from build123d import *

# Parameters (mm, degrees)
BOSS_EXTRUDE1_DEPTH = 4
SKETCH2_R           = 2
SKETCH2_R_2         = 1.5
CUT_EXTRUDE1_DEPTH  = 95.026591983
SKETCH4_W           = 20
SKETCH4_H           = 100
BOSS_EXTRUDE2_DEPTH = 4
FILLET3_R           = 42
FILLET4_R           = 12
SKETCH7_R           = 2
CUT_EXTRUDE3_DEPTH  = 105.120122935
CHAMFER1_SIZE       = 10
FILLET8_R           = 2
CUT_EXTRUDE4_DEPTH  = 105.120122935
CUT_EXTRUDE5_DEPTH  = 105.120122935
SKETCH10_W          = 4
SKETCH10_H          = 14.148423286
CUT_EXTRUDE6_DEPTH  = 105.120122935
FILLET11_R          = 3
FILLET12_R          = 3


with BuildPart() as part:
    # Sketch1 → Boss-Extrude1 (new body)
    with BuildSketch(Plane.XY):
        Polygon((-40, 60), (-25, 60), (-25, 52), (-15, 52), (-15, 0), (-21, 0), (-21, -50), (21, -50), (21, 0), (15, 0), (15, 52), (25, 52), (25, 60), (40, 60), (40, -60), (22, -60), (22, -85), (12, -85), (12, -60), (-12, -60), (-12, -85), (-22, -85), (-22, -60), (-40, -60), align=None)
    extrude(amount=BOSS_EXTRUDE1_DEPTH)

    # Sketch2 → Cut-Extrude1 (cut, through all)
    with BuildSketch(Plane(origin=(0, 0, 0), x_dir=(-1, 0, 0), z_dir=(0, 0, -1))):
        with Locations((-28.5, -32)):
            Circle(SKETCH2_R)
        with Locations((17, -56.5)):
            Circle(SKETCH2_R_2)
        with Locations((28.8, -32)):
            Circle(SKETCH2_R)
        with Locations((-17, -56.5)):
            Circle(SKETCH2_R_2)
    extrude(amount=-CUT_EXTRUDE1_DEPTH, mode=Mode.SUBTRACT)

    # Sketch4 → Boss-Extrude2 (add)
    with BuildSketch(Plane.XY.offset(4)):
        with Locations((-50, 10)):
            Rectangle(SKETCH4_W, SKETCH4_H)
        with Locations((50, 10)):
            Rectangle(SKETCH4_W, SKETCH4_H)
    extrude(amount=-BOSS_EXTRUDE2_DEPTH)

    # Fillet3
    # the kernel refuses this fillet: 42 mm, written as the material it takes off along each edge
    with BuildSketch(Plane(origin=(60, 60, 107.531396204), x_dir=(0, -1, 0), z_dir=(0, 0, -1))) as fillet3_piece_1:
        with BuildLine():
            CenterArc((41.412558482, 42), FILLET3_R, 189.594068227, 80.405931773)
            Line((0, 35), (-0.82825117, 34.86))
            ThreePointArc((-0.82825117, 34.86), (-0.84, 17.5), (-0.84, 0))
            Line((-0.84, 0), (0, -0.84))
            Line((0, -0.84), (41.412558482, -0.84))
            Line((41.412558482, -0.84), (41.412558482, 0))
        make_face()
    extrude(amount=211.062792409, mode=Mode.SUBTRACT)
    with BuildSketch(Plane(origin=(-60, 60, 107.531396204), x_dir=(1, 0, 0), z_dir=(0, 0, -1))) as fillet3_piece_2:
        with BuildLine():
            CenterArc((42, 41.412558482), FILLET3_R, 180, 80.405931773)
            Line((0, 41.412558482), (-0.84, 41.412558482))
            Line((-0.84, 41.412558482), (-0.84, 0))
            Line((-0.84, 0), (0, -0.84))
            ThreePointArc((0, -0.84), (17.5, -0.84), (34.86, -0.82825117))
            Line((34.86, -0.82825117), (35, 0))
        make_face()
    extrude(amount=211.062792409, mode=Mode.SUBTRACT)

    # Fillet4
    fillet4_edges = [part.edges().sort_by_distance(p)[0] for p in [
        (60, -40, 2),
        (-60, -40, 2),
    ]]
    fillet(fillet4_edges, radius=FILLET4_R)

    # Sketch7 → Cut-Extrude3 (cut, through all)
    with BuildSketch(Plane.XY):
        with Locations(Location((-55, -20, 0), (0, 0, 180))):
            Circle(SKETCH7_R)
        with Locations(Location((55, -20, 0), (0, 0, 180))):
            Circle(SKETCH7_R)
        with Locations(Location((-37, -20, 0), (0, 0, 180))):
            Circle(SKETCH7_R)
        with Locations(Location((37, -20, 0), (0, 0, 180))):
            Circle(SKETCH7_R)
    extrude(amount=CUT_EXTRUDE3_DEPTH, mode=Mode.SUBTRACT)

    # Chamfer1
    chamfer1_edges = [part.edges().sort_by_distance(p)[0] for p in [
        (-40, -60, 2),
        (40, -60, 2),
    ]]
    chamfer(chamfer1_edges, length=CHAMFER1_SIZE)

    # Fillet8
    fillet8_edges = [part.edges().sort_by_distance(p)[0] for p in [
        (-30, -60, 2),
        (-40, -50, 2),
        (30, -60, 2),
        (40, -50, 2),
        (40, -40, 2),
        (-40, -40, 2),
    ]]
    fillet(fillet8_edges, radius=FILLET8_R)

    # Sketch8 → Cut-Extrude4 (cut, through all)
    with BuildSketch(Plane(origin=(0, 0, 0), x_dir=(-1, 0, 0), z_dir=(0, 0, -1))):
        with BuildLine():
            ThreePointArc((-17.964817996, 17.438774634), (-30.770630407, 21.535466224), (-44.214817996, 21.375674028))
            ThreePointArc((-44.214817996, 21.375674028), (-45.841525426, 19.061841075), (-43.527692473, 17.435133644))
            ThreePointArc((-43.527692473, 17.435133644), (-31.363903701, 17.579707536), (-19.777692473, 13.87317705))
            ThreePointArc((-19.777692473, 13.87317705), (-17.088456442, 14.749538603), (-17.964817996, 17.438774634))
        make_face()
        with BuildLine():
            ThreePointArc((17.964817996, 17.438774634), (30.770630407, 21.535466224), (44.214817996, 21.375674028))
            ThreePointArc((44.214817996, 21.375674028), (45.841525426, 19.061841075), (43.527692473, 17.435133644))
            ThreePointArc((43.527692473, 17.435133644), (31.363903701, 17.579707536), (19.777692473, 13.87317705))
            ThreePointArc((19.777692473, 13.87317705), (17.088456442, 14.749538603), (17.964817996, 17.438774634))
        make_face()
    extrude(amount=-CUT_EXTRUDE4_DEPTH, mode=Mode.SUBTRACT)

    # Sketch9 → Cut-Extrude5 (cut, through all)
    with BuildSketch(Plane.XY.offset(4)):
        Polygon((-24, 52), (-20, 52), (-20, 45.2), (-18.25, 45.2), (-18.25, 42), (-25.75, 42), (-25.75, 45.2), (-24, 45.2), align=None)
    cut_extrude5 = extrude(amount=-CUT_EXTRUDE5_DEPTH, mode=Mode.SUBTRACT)

    # Mirror1: Cut-Extrude5 across plane
    add(cut_extrude5.mirror(Plane(origin=(0, 0, 0), x_dir=(0, 0, 1), z_dir=(1, 0, 0))), mode=Mode.SUBTRACT)

    # Sketch10 → Cut-Extrude6 (cut, through all)
    with BuildSketch(Plane.XY.offset(4)):
        with Locations((46, -32.925788357)):
            Rectangle(SKETCH10_W, SKETCH10_H)
        with BuildLine():
            Line((44, -19.851576714), (48, -19.851576714))
            Line((48, -19.851576714), (48, -3.703153428))
            Line((48, -3.703153428), (56.485281374, -3.703153428))
            Line((56.485281374, -3.703153428), (53.762388988, 27.211478811))
            Line((53.762388988, 27.211478811), (53.006446404, 28.506843132))
            Line((53.006446404, 28.506843132), (57.992638284, 31.416661411))
            ThreePointArc((57.992638284, 31.416661411), (47.696624216, 48.287786805), (30.824208916, 58.581686925))
            Line((30.824208916, 58.581686925), (49.856368895, 25.968653244))
            Line((49.856368895, 25.968653244), (52.117484809, 0.296846572))
            Line((52.117484809, 0.296846572), (44, 0.296846572))
            Line((44, 0.296846572), (44, -19.851576714))
        make_face()
    cut_extrude6 = extrude(amount=-CUT_EXTRUDE6_DEPTH, mode=Mode.SUBTRACT)

    # Mirror5: Cut-Extrude6 across plane
    add(cut_extrude6.mirror(Plane(origin=(0, 0, 0), x_dir=(0, 0, 1), z_dir=(1, 0, 0))), mode=Mode.SUBTRACT)

    # Fillet11
    fillet11_edges = [part.edges().sort_by_distance(p)[0] for p in [
        (-53.762388988, 27.211478811, 2),
        (-49.856368895, 25.968653244, 2),
        (-52.117484809, 0.296846572, 2),
        (-56.485281374, -3.703153428, 2),
        (-48, -3.703153428, 2),
        (-44, 0.296846572, 2),
        (-48, -40, 2),
        (-44, -40, 2),
        (53.762388988, 27.211478811, 2),
        (49.856368895, 25.968653244, 2),
        (52.117484809, 0.296846572, 2),
        (56.485281374, -3.703153428, 2),
        (48, -3.703153428, 2),
        (44, 0.296846572, 2),
        (44, -40, 2),
        (48, -40, 2),
    ]]
    fillet(fillet11_edges, radius=FILLET11_R)

    # Fillet12
    fillet12_edges = [part.edges().sort_by_distance(p)[0] for p in [
        (-53.006446404, 28.506843132, 2),
        (53.006446404, 28.506843132, 2),
    ]]
    fillet(fillet12_edges, radius=FILLET12_R)


solid = part.part
Input: part model. Units: mm. Frame: model coordinates. A direction names the side the tool comes from. Coordinates: 2 decimals unless noted, no trailing zeros. Order: outer loops, then holes, each group sorted by start corner. A loop starts at its lowest first (then second) coordinate and runs counter-clockwise, first axis right, second up. Notation, with made-up numbers: M 2.25,-24 L 27.25,-24 A22 ccw 27.25,4 Z; hole C 19.25,7.25 d2. An arc over 180 degrees is marked long. Answer in a Markdown table with one row per item.
(1) Section query B-B, the plane x = -32.5. Output: boundary loops of the cut face in (y, z).
Numbers:
| item | result |
|---|---|
| outline | M -57.5,0 L 17.73,0 L 17.73,4 L -57.5,4 Z; M 21.76,0 L 55.71,0 L 55.71,4 L 21.76,4 Z |
(2) Section query D-D, the plane x = -5.5. Output: boundary loops of the cut face in (y, z), plus the area to 3 significant figures.
Numbers:
| item | result |
|---|---|
| outline | M -60,0 L -50,0 L -50,4 L -60,4 Z |
| area | 40.0 mm^2 |
(3) Draft query along X for faces 1 (the flat face through (17, -85, 2)), 2 (the flat face through (35, -55, 2)), 3 (the flat face through (-48, -13, 2)), 4 (the flat face through (-15, 26, 2)). Return one class per face: pulls with the +X half, pulls with the -X half, needs draft (parallel to the pull), parting line crosses it, or undercut.
Numbers:
| item | result |
|---|---|
| face 1 | needs draft |
| face 2 | pulls with the +X half |
| face 3 | undercut |
| face 4 | undercut |
(4) Section query A-A, the plane y = -67. Output: boundary loops of the cut face in (x, z), plus the area to 3 significant figures.
Numbers:
| item | result |
|---|---|
| outline | M -22,0 L -12,0 L -12,4 L -22,4 Z; M 12,0 L 22,0 L 22,4 L 12,4 Z |
| area | 80.0 mm^2 |
(5) Section query C-C, the plane y = -32. Output: boundary loops of the cut face in (x, z), plus the area to 3 significant figures.
Numbers:
| item | result |
|---|---|
| outline | M -59.31,0 L -48,0 L -48,4 L -59.31,4 Z; M -44,0 L -30.8,0 L -30.8,4 L -44,4 Z; M -26.8,0 L -21,0 L -21,4 L -26.8,4 Z; M 21,0 L 26.5,0 L 26.5,4 L 21,4 Z; M 30.5,0 L 44,0 L 44,4 L 30.5,4 Z; M 48,0 L 59.31,0 L 59.31,4 L 48,4 Z |
| area | 243 mm^2 |
(6) Material intervals for line 1 (Y direction, x = -37, z = 1); line 2 (X direction, y = -20, z = 2.65); line 3 (X direction, y = -71, z = 2.65), sorted ascending. Write a range as [from, to].
Numbers:
| item | result |
|---|---|
| line 1 | y = [-53, -22], [-18, 18], [22, 48] |
| line 2 | x = [-60, -57], [-53, -39], [-35, -21], [21, 35], [39, 53], [57, 60] |
| line 3 | x = [-22, -12], [12, 22] |
(7) Contact query for flat-ended pins moving along their axis: pin 1 Ø1.4 at (x, z) = (24.5, 2.5) entering from -Y; pin 2 Ø2 at (y, z) = (41.5, 3.5) entering from +X; pin 3 Ø1 at (y, z) = (-45, 3.5) entering from +X; pin 4 Ø6.5 at (x, y) = (37, -20) entering from +Z. Output: stop coordinate, or through.
Numbers:
| item | result |
|---|---|
| pin 1 | stops at y = -60 |
| pin 2 | stops at x = 41.38 |
| pin 3 | stops at x = 40 |
| pin 4 | stops at z = 4 |
(8) Access query for faces 5 (the cylindrical face through (31.5, 17.6, 2)), 6 (the cylindrical face through (27.897, 59.405, 2.028)), 7 (the flat face through (25, 56, 2)), 8 (the flat face through (-22, -73, 2)). Directions: +Z, -Z, +X, -X, +Y, -Y. A direction counts if a zero-diameter tool reaches every point of the face in a straight line with its end or side. Return the directions, or none.
Numbers:
| item | result |
|---|---|
| face 5 | +Z, -Z |
| face 6 | +Z, -Z, +X, +Y |
| face 7 | +Z, -Z, +Y |
| face 8 | +Z, -Z, -X, -Y |
